```python
from build123d import *

# Parameters (mm, degrees)
BOSS_EXTRUDE1_DEPTH   = 0.8
BOSS_EXTRUDE2_DEPTH   = 1.3
BOSS_EXTRUDE3_DEPTH   = 0.9
BOSS_EXTRUDE3_TAPER   = 10
SKETCH4_R             = 1.6
SKETCH4_R_2           = 0.9
BOSS_EXTRUDE4_DEPTH   = 2.65
SKETCH5_R             = 0.6
BOSS_EXTRUDE5_DEPTH   = 3
CHAMFER1_SIZE         = 0.5
CHAMFER1_SIZE2        = 0.419549816
CHAMFER1_PART_2_SIZE  = 0.5
CHAMFER1_PART_2_SIZE2 = 0.419549816
CHAMFER1_PART_3_SIZE  = 0.5
CHAMFER1_PART_3_SIZE2 = 0.419549816
CHAMFER2_SIZE         = 0.5
SKETCH6_W             = 16.5
SKETCH6_H             = 17.5
BOSS_EXTRUDE6_DEPTH   = 4
CHAMFER3_SIZE         = 2.5
CHAMFER3_SIZE2        = 0.669872981
CHAMFER4_SIZE         = 2.5
CHAMFER4_SIZE2        = 1.165769145
CHAMFER4_PART_2_SIZE  = 2.5
CHAMFER4_PART_2_SIZE2 = 1.165769145
CHAMFER5_SIZE         = 2.5


with BuildPart() as part:
    # Sketch1 → Boss-Extrude1 (new body)
    with BuildSketch(Plane(origin=(0, 0, 0), x_dir=(1, 0, 0), z_dir=(0, 1, 0))):
        with BuildLine():
            Line((-6.5, -7.5), (6.5, -7.5))
            ThreePointArc((6.5, -7.5), (7.207106781, -7.207106781), (7.5, -6.5))
            Line((7.5, -6.5), (7.5, 6.5))
            ThreePointArc((7.5, 6.5), (7.207106781, 7.207106781), (6.5, 7.5))
            Line((6.5, 7.5), (-6.5, 7.5))
            ThreePointArc((-6.5, 7.5), (-7.207106781, 7.207106781), (-7.5, 6.5))
            Line((-7.5, 6.5), (-7.5, -6.5))
            ThreePointArc((-7.5, -6.5), (-7.207106781, -7.207106781), (-6.5, -7.5))
        make_face()
    extrude(amount=BOSS_EXTRUDE1_DEPTH)

    # Sketch2 → Boss-Extrude2 (add)
    with BuildSketch(Plane.XZ):
        with BuildLine():
            Line((-6.9, 6.5), (-6.9, -6.5))
            ThreePointArc((-6.9, -6.5), (-6.782842712, -6.782842712), (-6.5, -6.9))
            Line((-6.5, -6.9), (6.5, -6.9))
            ThreePointArc((6.5, -6.9), (6.782842712, -6.782842712), (6.9, -6.5))
            Line((6.9, -6.5), (6.9, 6.5))
            ThreePointArc((6.9, 6.5), (6.782842712, 6.782842712), (6.5, 6.9))
            Line((6.5, 6.9), (-6.5, 6.9))
            ThreePointArc((-6.5, 6.9), (-6.782842712, 6.782842712), (-6.9, 6.5))
        make_face()
    extrude(amount=BOSS_EXTRUDE2_DEPTH)

    # Sketch3 → Boss-Extrude3 (add)
    with BuildSketch(Plane.XZ.offset(1.3)):
        with BuildLine():
            Line((-6.9, 6.5), (-6.9, -6.5))
            ThreePointArc((-6.9, -6.5), (-6.782842712, -6.782842712), (-6.5, -6.9))
            Line((-6.5, -6.9), (6.5, -6.9))
            ThreePointArc((6.5, -6.9), (6.782842712, -6.782842712), (6.9, -6.5))
            Line((6.9, -6.5), (6.9, 6.5))
            ThreePointArc((6.9, 6.5), (6.782842712, 6.782842712), (6.5, 6.9))
            Line((6.5, 6.9), (-6.5, 6.9))
            ThreePointArc((-6.5, 6.9), (-6.782842712, 6.782842712), (-6.9, 6.5))
        make_face()
    extrude(amount=BOSS_EXTRUDE3_DEPTH, taper=BOSS_EXTRUDE3_TAPER)

    # Sketch4 → Boss-Extrude4 (add)
    with BuildSketch(Plane.XZ.offset(2.2)):
        Circle(SKETCH4_R)
        with Locations((0, -5.5)):
            Circle(SKETCH4_R_2)
        with Locations((0, 5.5)):
            Circle(SKETCH4_R_2)
    extrude(amount=BOSS_EXTRUDE4_DEPTH)

    # Sketch5 → Boss-Extrude5 (add)
    with BuildSketch(Plane.XZ.offset(2.2)):
        with Locations((-5.9, 0)):
            Circle(SKETCH5_R)
        with Locations((-3.8, -5)):
            Circle(SKETCH5_R)
        with Locations((-3.8, 5)):
            Circle(SKETCH5_R)
    extrude(amount=BOSS_EXTRUDE5_DEPTH)

    # Chamfer1
    chamfer1_edges = [part.edges().sort_by_distance(p)[0] for p in [
        (-6.5, -5.2, 0),
    ]]
    chamfer1_side = [part.faces().sort_by_distance(p)[0] for p in [
        (-6.5, -3.7, 0),
    ]]
    chamfer(chamfer1_edges, length=CHAMFER1_SIZE, length2=CHAMFER1_SIZE2, reference=chamfer1_side[0])

    # Chamfer1 part 2
    chamfer1_part_2_edges = [part.edges().sort_by_distance(p)[0] for p in [
        (-4.4, -5.2, -5),
    ]]
    chamfer1_part_2_side = [part.faces().sort_by_distance(p)[0] for p in [
        (-4.4, -3.7, -5),
    ]]
    chamfer(chamfer1_part_2_edges, length=CHAMFER1_PART_2_SIZE, length2=CHAMFER1_PART_2_SIZE2, reference=chamfer1_part_2_side[0])

    # Chamfer1 part 3
    chamfer1_part_3_edges = [part.edges().sort_by_distance(p)[0] for p in [
        (-4.4, -5.2, 5),
    ]]
    chamfer1_part_3_side = [part.faces().sort_by_distance(p)[0] for p in [
        (-4.4, -3.7, 5),
    ]]
    chamfer(chamfer1_part_3_edges, length=CHAMFER1_PART_3_SIZE, length2=CHAMFER1_PART_3_SIZE2, reference=chamfer1_part_3_side[0])

    # Chamfer2
    chamfer2_edges = [part.edges().sort_by_distance(p)[0] for p in [
        (-1.6, -4.85, 0),
        (-0.9, -4.85, -5.5),
        (-0.9, -4.85, 5.5),
    ]]
    chamfer(chamfer2_edges, length=CHAMFER2_SIZE)

    # Sketch6 → Boss-Extrude6 (add)
    with BuildSketch(Plane(origin=(0, 0.8, 0), x_dir=(1, 0, 0), z_dir=(0, 1, 0))):
        Rectangle(SKETCH6_W, SKETCH6_H)
    extrude(amount=BOSS_EXTRUDE6_DEPTH)

    # Chamfer3
    chamfer3_edges = [part.edges().sort_by_distance(p)[0] for p in [
        (8.25, 4.8, 0),
    ]]
    chamfer3_side = [part.faces().sort_by_distance(p)[0] for p in [
        (8.25, 2.8, 0),
    ]]
    chamfer(chamfer3_edges, length=CHAMFER3_SIZE, length2=CHAMFER3_SIZE2, reference=chamfer3_side[0])

    # Chamfer4
    chamfer4_edges = [part.edges().sort_by_distance(p)[0] for p in [
        (-0.334936491, 4.8, -8.75),
    ]]
    chamfer4_side = [part.faces().sort_by_distance(p)[0] for p in [
        (-0.103143341, 2.785008314, -8.75),
    ]]
    chamfer(chamfer4_edges, length=CHAMFER4_SIZE, length2=CHAMFER4_SIZE2, reference=chamfer4_side[0])

    # Chamfer4 part 2
    chamfer4_part_2_edges = [part.edges().sort_by_distance(p)[0] for p in [
        (-0.334936491, 4.8, 8.75),
    ]]
    chamfer4_part_2_side = [part.faces().sort_by_distance(p)[0] for p in [
        (-0.103143341, 2.785008314, 8.75),
    ]]
    chamfer(chamfer4_part_2_edges, length=CHAMFER4_PART_2_SIZE, length2=CHAMFER4_PART_2_SIZE2, reference=chamfer4_part_2_side[0])

    # Chamfer5
    chamfer5_edges = [part.edges().sort_by_distance(p)[0] for p in [
        (-8.25, 4.8, 0),
    ]]
    chamfer(chamfer5_edges, length=CHAMFER5_SIZE)


solid = part.part
```
Input: part model. Units: mm. Frame: model coordinates. A direction names the side the tool comes from. Give positions to 0.01 mm unless a question says otherwise; leave off trailing zeros. Order: outer loops, then holes, each group sorted by start corner. A loop starts at its lowest first (then second) coordinate and runs counter-clockwise, first axis right, second up. Notation, with made-up numbers: (24, -19) -> (35, -19) arc R22 ccw to (35, 12) -> close; hole circle Ø3 at (87, 23). An arc over 180 degrees is marked (long way). Write each question's results on one line, items separated by ' | '. Start each with the question number.
Item 1: Line query: line 1 (Y direction, x = -1.25, z = -5.75); line 2 (X direction, y = -0.5, z = 6); line 3 (Y direction, x = -1, z = 7). Output: solid intervals per line, ascending.
Item 2: Cut plane B-B on y = 3. Return the cut outline in (x, z).
Item 3: Mould query, pull axis Z, two halves, no side actions, for faces 5 (the cylindrical face through (-3.93, -3.432, 4.414)), 6 (the cylindrical face through (-1.27, -3.26, -0.97)), 7 (the cylindrical face through (7.215, 0.394, -7.199)), 8 (the flat face through (0, -4.85, 0)). Classes: pulls with the +Z half, pulls with the -Z half, needs draft (parallel to the pull), parting line crosses it, or undercut.
Item 4: Set-up query: faces 1 (the flat face through (6.9, -1, 0)), 2 (the cylindrical face through (-7.215, 0.394, 7.199)), 3 (the cylindrical face through (-6.5, -3.4, 0)), 4 (the flat face through (0, -1, -6.9)). Return all of +Z, -Z, +X, -X, +Y, -Y with unobstructed straight access to the full face (end or side cutting, diameter ignored); none if empty.
Item 5: Contact query for flat-ended pins moving along their axis: P1, Ø2.5, axis at x = 0, z = -0.5, coming from the -Y side; P2, Ø2, axis at x = 1.5, z = 2, coming from the -Y side; P3, Ø1, axis at x = 3, y = -1, coming from the -Z side. Output: stop coordinate, or through.
Item 6: Cut plane A-A on y = -3. Return the cut outline in (x, z), then the cut area to 3 significant figures.
Established:
1) line 1: -2.2 to 4.8 | line 2: -6.9 to 6.9 | line 3: 0 to 4.8
2) outline: (-7.55, -8.42) -> (8.06, -8.42) -> (8.06, 8.42) -> (-7.55, 8.42) -> close
3) face 5: undercut | face 6: undercut | face 7: pulls with the -Z half | face 8: needs draft
4) face 1: +Z, -Z, +X, -Y | face 2: +Z, -X, -Y | face 3: -Y | face 4: -Z, +X, -X, -Y
5) P1: y = -4.85 | P2: y = -4.45 | P3: z = -6.9
6) outline: circle Ø1.2 at (-5.9, 0); circle Ø1.2 at (-3.8, -5); circle Ø1.2 at (-3.8, 5); circle Ø3.2 at (0, 0); circle Ø1.8 at (0, -5.5); circle Ø1.8 at (0, 5.5) | area: 16.5 mm^2
